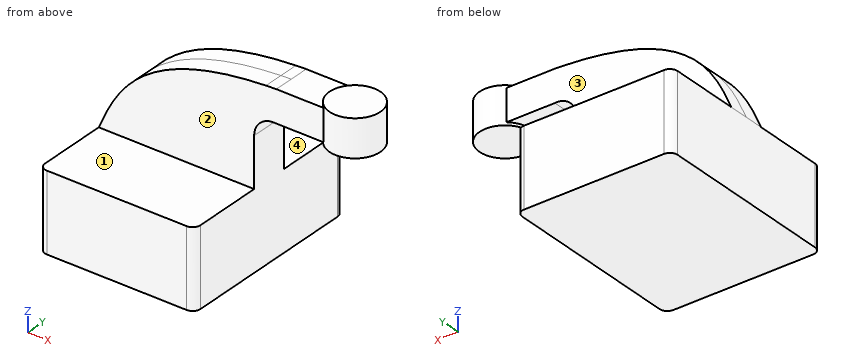
```python
from build123d import *

# Parameters (mm, degrees)
F1_DEPTH = 63.5
F0_W     = 17.5679588894
F0_H     = 20.8251091272
F2_DEPTH = 12.7
F4_R     = 5.08
F5_R     = 5.08


with BuildPart() as f1:
    # F0 (on Front) → F1 (new body, symmetric)
    with BuildSketch(Plane.XZ):
        Polygon((-50.8, 25.4), (-50.8, -25.4), (50.8, -25.4), (50.8, 25.4), (29.9748908728, 25.4), align=None)
    extrude(amount=F1_DEPTH, both=True)

    # F0 (on Front) → F2 (join, symmetric)
    with BuildSketch(Plane.XZ):
        with BuildLine():
            add(Edge.make_bspline(
                [(-50.8, 25.4), (-40.0576822889, 49.6242242179), (-26.1354784037, 86.069146105), (58.5620329332, 90.9465027441)],
                knots=[0, 0, 0, 0, 130.1130965779, 130.1130965779, 130.1130965779, 130.1130965779], degree=3))
            Line((-50.8, 25.4), (29.9748908728, 25.4))
            Line((29.9748908728, 25.4), (29.9748908728, 57.7870482366))
            ThreePointArc((29.9748908728, 57.7870482366), (38.1082806139, 79.6775376922), (58.5620329332, 90.9465027441))
        make_face()
        with BuildLine():
            Line((29.9748908728, 25.4), (50.8, 25.4))
            Line((50.8, 25.4), (50.8, 57.7870482366))
            ThreePointArc((50.8, 57.7870482366), (54.9254885829, 67.1554928224), (64.6216935366, 70.4374159629))
            Line((64.6216935366, 70.4374159629), (89.3876225336, 70.4374159629))
            Line((89.3876225336, 70.4374159629), (89.3876225336, 91.2625250901))
            Line((89.3876225336, 91.2625250901), (65.3235655796, 91.2625250901))
            add(Edge.make_bspline(
                [(58.5620329332, 90.9465027441), (60.7674907461, 91.0735053459), (63.0209371473, 91.1791038317), (65.3235655796, 91.2625250901)],
                knots=[130.1130965779, 130.1130965779, 130.1130965779, 130.1130965779, 133.5011411718, 133.5011411718, 133.5011411718, 133.5011411718], degree=3))
            ThreePointArc((58.5620329332, 90.9465027441), (38.1082806139, 79.6775376922), (29.9748908728, 57.7870482366))
            Line((29.9748908728, 57.7870482366), (29.9748908728, 25.4))
        make_face()
        with Locations((98.1716019783, 80.8499705265)):
            Rectangle(F0_W, F0_H)
    extrude(amount=F2_DEPTH, both=True)

    # F0 (on Front) → F3 (revolve)
    with BuildSketch(Plane.XZ):
        Polygon((106.955581423, 92.8989347667), (106.955581423, 91.2625250901), (106.955581423, 70.4374159629), (106.955581423, 68.5675365603), (123.5830926897, 68.5675365603), (123.5830926897, 92.8989347667), align=None)
    revolve(axis=Axis((106.955581423, 0, 80.7332356635), (0, 0, -1)))

    # F4
    f4_edges = [f1.edges().sort_by_distance(p)[0] for p in [
        (50.8, -63.5, 0),
        (-50.8, -63.5, 0),
        (50.8, 63.5, 0),
    ]]
    fillet(f4_edges, radius=F4_R)

    # F5
    f5_edges = [f1.edges().sort_by_distance(p)[0] for p in [
        (-50.8, 63.5, 0),
    ]]
    fillet(f5_edges, radius=F5_R)


solid = f1.part
```
The listing builds one solid part. Answer for the finished solid, in the listing's coordinates (mm). Face numbers are marked on the shaded views. A direction names the side the tool comes from. Give positions to 0.01 mm unless a question says otherwise; leave off trailing zeros. Loops run counter-clockwise (first coordinate to the right, second up) from the corner with the lowest first, then second, coordinate; pieces in that order, holes last. Notation, with made-up numbers: (-34, 41) - (-4, 41) arc R21 cw to (-4, 62) - close; hole circle Ø10 at (13, 64). An arc over 180 degrees is marked (long way). Return JSON: item names as keys, results as strings. Group by question number.
1. Which of the six approach directions +Z, -Z, +X, -X, +Y, -Y give full straight-line access (tool end or side, diameter ignored) to the marked faces 1, 2, 3 and 4?
2. Find section A-A (x = 78). Write down the section's boundary in (y, z).
3. Straight lines are drawn through the part: line 1 (X direction, y = 24, z = 9); line 2 (Z direction, x = 102, y = 10); line 3 (Z direction, x = -33.5, y = -48.5). For each, find the intervals that lie inside material, in ascending order. Write a range as [from, to].
4. Given pin 1 Ø12.5 at (x, y) = (87, -3) entering from +Z; pin 2 Ø3 at (x, y) = (63.5, 5) entering from -Z; pin 3 Ø6 at (y, z) = (-1, 32.5) entering from +X; pin 4 Ø10 at (x, y) = (40.5, -45) entering from +Z, each flat-ended and moving along its own axis, determine where each tip first touches the part or whether it passes through.
5. Find section B-B (y = -50.5). Write down the section's boundary in (x, z).
Verdict:
{
 "1": {"face 1": "+Z, +X, -X, -Y", "face 2": "+Z, -X, -Y", "face 3": "+Z, -X, +Y", "face 4": "+Z, +X, -X, +Y"},
 "2": {"outline": "(-12.7, 70.44) - (12.7, 70.44) - (12.7, 91.26) - (-12.7, 91.26) - close"},
 "3": {"line 1": "x = [-50.8, 50.8]", "line 2": "z = [68.57, 92.9]", "line 3": "z = [-25.4, 25.4]"},
 "4": {"pin 1": "stops at z = 92.9", "pin 2": "stops at z = 70.4", "pin 3": "stops at x = 50.8", "pin 4": "stops at z = 25.4"},
 "5": {"outline": "(-50.8, -25.4) - (50.8, -25.4) - (50.8, 25.4) - (-50.8, 25.4) - close"}
}
